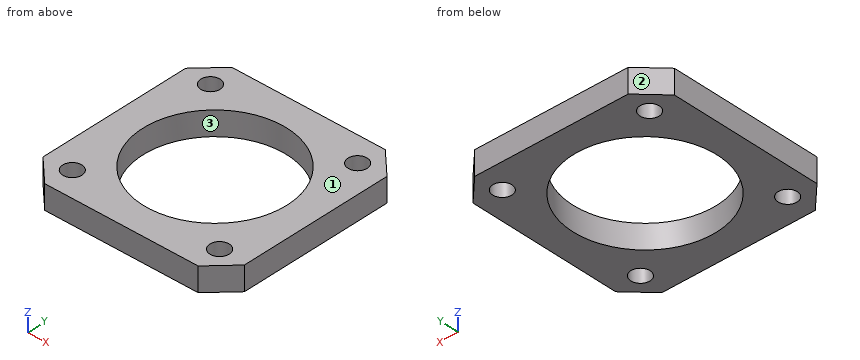
from build123d import *

# Parameters (mm, degrees)
SKETCH1_W           = 42
SKETCH1_H           = 42
BOSS_EXTRUDE1_DEPTH = 5
SKETCH2_R           = 15
CUT_EXTRUDE1_DEPTH  = 6
SKETCH4_R           = 2
CUT_EXTRUDE3_DEPTH  = 5
CHAMFER1_SIZE       = 5


with BuildPart() as part:
    # Sketch1 → Boss-Extrude1 (new body)
    with BuildSketch(Plane.XY):
        with Locations((21, 21)):
            Rectangle(SKETCH1_W, SKETCH1_H)
    extrude(amount=BOSS_EXTRUDE1_DEPTH)

    # Sketch2 → Cut-Extrude1 (cut, through all)
    with BuildSketch(Plane.XY.offset(5)):
        with Locations((21, 21)):
            Circle(SKETCH2_R)
    extrude(amount=-CUT_EXTRUDE1_DEPTH, mode=Mode.SUBTRACT)

    # Sketch4 → Cut-Extrude3 (cut)
    with BuildSketch(Plane.XY.offset(5)):
        with Locations((5.65, 36.5)):
            Circle(SKETCH4_R)
        with Locations((5.65, 5.5)):
            Circle(SKETCH4_R)
        with Locations((36.35, 5.5)):
            Circle(SKETCH4_R)
        with Locations((36.35, 36.5)):
            Circle(SKETCH4_R)
    extrude(amount=-CUT_EXTRUDE3_DEPTH, mode=Mode.SUBTRACT)

    # Chamfer1
    chamfer1_edges = [part.edges().sort_by_distance(p)[0] for p in [
        (0, 42, 2.5),
        (42, 42, 2.5),
        (42, 0, 2.5),
        (0, 0, 2.5),
    ]]
    chamfer(chamfer1_edges, length=CHAMFER1_SIZE)


solid = part.part
Could you check a few things on this model? Use its own coordinates, in mm. Face numbers are marked on the shaded views. Give positions to 0.01 mm unless a question says otherwise; leave off trailing zeros. Order: outer loops, then holes, each group sorted by start corner. A loop starts at its lowest first (then second) coordinate and runs counter-clockwise, first axis right, second up. Notation, with made-up numbers: (75, -39.75) - (113, -39.75) arc R25 cw to (113, -7.75) - close; hole circle Ø8 at (89, 89). An arc over 180 degrees is marked (long way). Return JSON: item names as keys, results as strings. Group by question number.
Q1. Will this pin go through, and if not, where does the flat tip stop? pin 1 Ø2.5 at (x, y) = (36.35, 5.5) entering from +Z.
Q2. Please list where these lines run through material, in increasing order: line 1 along Y through (x, z) = (5.65, 1.5); line 2 along X through (y, z) = (5, 4.4); line 3 along Y through (x, z) = (21, 3.9). Write a range as [from, to].
Q3. Suppose I cut it at B-B, the plane x = 15. Please give me the cut outline in (y, z).
Q4. Suppose I cut it at A-A, the plane y = 12. Please give me the cut outline in (x, z).
Q5. Suppose I cut it at D-D, the plane y = 5.5. Please give me the cut outline in (x, z).
Q6. Suppose I cut it at C-C, the plane z = 4.4. Please give me the cut outline in (x, y), and give its area (3 significant figures).
Q7. Thinking about a two-plate mould opening in Y: for the marked faces 1, 2 and 3, which applies, pulls with the +Y half, pulls with the -Y half, needs draft (parallel to the pull), parting line crosses it, or undercut?
Resolved:
{
 "1": {"pin 1": "passes through"},
 "2": {"line 1": "y = [0, 3.5], [7.5, 34.5], [38.5, 42]", "line 2": "x = [0, 3.71], [7.59, 34.41], [38.29, 42]", "line 3": "y = [0, 6], [36, 42]"},
 "3": {"outline": "(0, 0) - (7.25, 0) - (7.25, 5) - (0, 5) - close; (34.75, 0) - (42, 0) - (42, 5) - (34.75, 5) - close"},
 "4": {"outline": "(0, 0) - (9, 0) - (9, 5) - (0, 5) - close; (33, 0) - (42, 0) - (42, 5) - (33, 5) - close"},
 "5": {"outline": "(0, 0) - (3.65, 0) - (3.65, 5) - (0, 5) - close; (7.65, 0) - (34.35, 0) - (34.35, 5) - (7.65, 5) - close; (38.35, 0) - (42, 0) - (42, 5) - (38.35, 5) - close"},
 "6": {"outline": "(0, 5) - (5, 0) - (37, 0) - (42, 5) - (42, 37) - (37, 42) - (5, 42) - (0, 37) - close; hole circle Ø4 at (5.65, 5.5); hole circle Ø4 at (5.65, 36.5); hole circle Ø30 at (21, 21); hole circle Ø4 at (36.35, 5.5); hole circle Ø4 at (36.35, 36.5)", "area": "957 mm2"},
 "7": {"face 1": "needs draft", "face 2": "pulls with the +Y half", "face 3": "undercut"}
}
